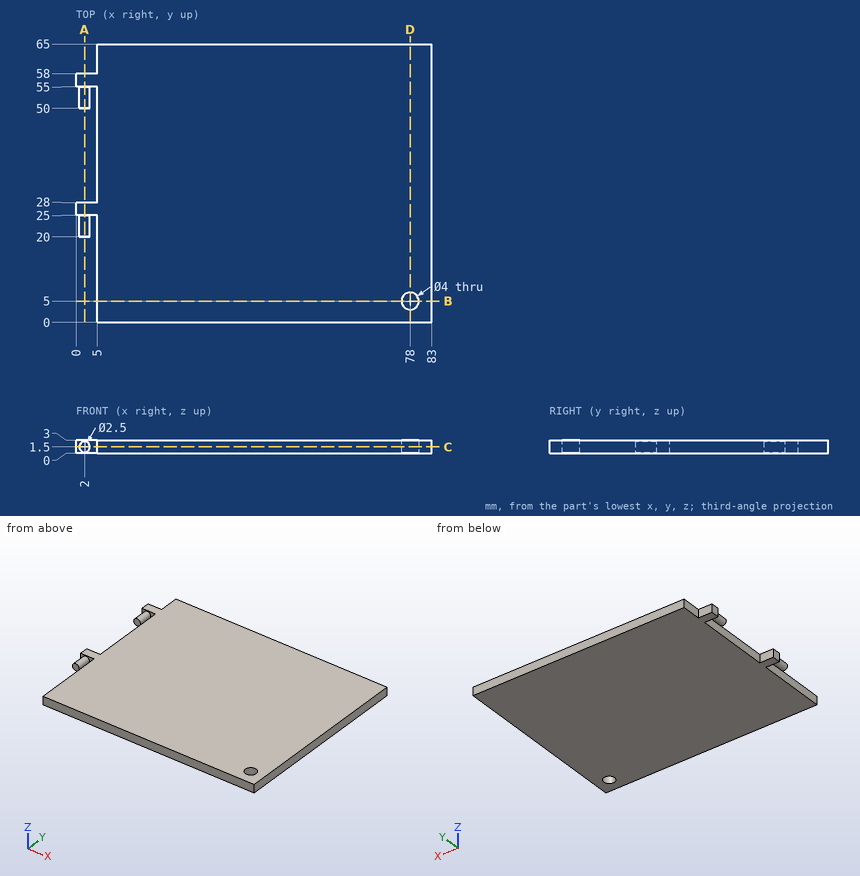
Drawing for the job (mm, zero at the part's lowest x, y, z). Round coordinates to 2 decimals unless told otherwise and drop trailing zeros. Write each loop counter-clockwise with the first axis right and the second up, starting at its lowest first coordinate (ties: lowest second). Pieces come first, ordered by that corner, then holes. Notation, with made-up numbers: (72, 6) - (104, 6) arc R14 ccw to (104, 29) - close; hole circle Ø8 at (63, 43.5). An arc over 180 degrees is marked (long way). Write item = value, one per line. Start each with the question number.
Q1. Drop flat-ended pins along their axis: pin 1 (1.5 mm diameter, centred on x = 1.5, z = 2, fed in from -Y); pin 2 (1.5 mm diameter, centred on y = 37.5, z = 1, fed in from -X); pin 3 (0.9 mm diameter, centred on x = 1.5, z = 2, fed in from +Y); pin 4 (2.5 mm diameter, centred on x = 78, y = 5, fed in from -Z). Give the stop position or say it passes through.
Q2. Band-saw the part on C-C (z = 1.5). Give the cut face in (x, y).
Q3. Band-saw the part on A-A (x = 2). Give the cut face in (y, z).
Q4. Band-saw the part on B-B (y = 5). Give the cut face in (x, z).
Q5. Probe L1, parallel to Y at x = 78, z = 0.85; L2, parallel to X at y = 42, z = 1.35; L3, parallel to X at y = 21.5, z = 1.95. List the from-to ranges inside material, lowest first. Write a range as from..to.
Q6. Band-saw the part on D-D (x = 78). Give the cut face in (y, z).
Answers below:
q1.pin_1 = 20
q1.pin_2 = 5
q1.pin_3 = 58
q1.pin_4 = through
q2.outline = (0, 25) - (0.75, 25) - (0.75, 20) - (3.25, 20) - (3.25, 25) - (5, 25) - (5, 0) - (83, 0) - (83, 65) - (5, 65) - (5, 58) - (0, 58) - (0, 55) - (0.75, 55) - (0.75, 50) - (3.25, 50) - (3.25, 55) - (5, 55) - (5, 28) - (0, 28) - close; hole circle Ø4 at (78, 5)
q3.outline = (20, 0.25) - (25, 0.25) - (25, 0) - (28, 0) - (28, 3) - (25, 3) - (25, 2.75) - (20, 2.75) - close; (50, 0.25) - (55, 0.25) - (55, 0) - (58, 0) - (58, 3) - (55, 3) - (55, 2.75) - (50, 2.75) - close
q4.outline = (5, 0) - (76, 0) - (76, 3) - (5, 3) - close; (80, 0) - (83, 0) - (83, 3) - (80, 3) - close
q5.L1 = 0..3, 7..65
q5.L2 = 5..83
q5.L3 = 0.83..3.17, 5..83
q6.outline = (0, 0) - (3, 0) - (3, 3) - (0, 3) - close; (7, 0) - (65, 0) - (65, 3) - (7, 3) - close
